```python
from build123d import *

# Parameters (mm, degrees)
SKETCH1_W                    = 50
SKETCH1_H                    = 150
BASE_FLANGE1_DEPTH           = 6
EDGE_FLANGE1_STRIP_W         = 36
EDGE_FLANGE1_STRIP_H         = 6
EDGE_FLANGE1_STRIP_CUT_DEPTH = 150
EDGE_FLANGE1_DEPTH           = 150
SKETCH9_R                    = 4
CUT_EXTRUDE1_DEPTH           = 6
CUT_EXTRUDE2_DEPTH           = 10
FILLET1_R                    = 5
SKETCH11_W                   = 20
SKETCH11_H                   = 80
SKETCH11_W_2                 = 70
SKETCH11_R                   = 4
SKETCH11_R_2                 = 20
CUT_EXTRUDE5_DEPTH           = 10


# Sheet-metal steps are written as plain solids
with BuildPart() as part:
    # Sketch1 → Base-Flange1 (new body)
    with BuildSketch(Plane.XY):
        with Locations((25, 75)):
            Rectangle(SKETCH1_W, SKETCH1_H)
    extrude(amount=-BASE_FLANGE1_DEPTH)

    # Edge-Flange1 strip (across the edge) → Edge-Flange1 strip cut (cut)
    with BuildSketch(Plane(origin=(50, 0, 0), x_dir=(-1, 0, 0), z_dir=(0, 1, 0))):
        with Locations((-6, -3)):
            Rectangle(EDGE_FLANGE1_STRIP_W, EDGE_FLANGE1_STRIP_H)
    extrude(amount=EDGE_FLANGE1_STRIP_CUT_DEPTH, mode=Mode.SUBTRACT)

    # Edge-Flange1 section (across the edge) → Edge-Flange1 (add)
    with BuildSketch(Plane(origin=(50, 0, 0), x_dir=(-1, 0, 0), z_dir=(0, 1, 0))):
        with BuildLine():
            Line((0, 6), (0, 144))
            Line((0, 144), (6, 144))
            Line((6, 144), (6, 6))
            ThreePointArc((6, 6), (7.757359313, 1.757359313), (12, 0))
            Line((12, 0), (12, -6))
            ThreePointArc((12, -6), (3.514718626, -2.485281374), (0, 6))
        make_face()
    extrude(amount=EDGE_FLANGE1_DEPTH)

    # Sketch9 → Cut-Extrude1 (cut)
    with BuildSketch(Plane.XY):
        with Locations((6.5, 135)):
            Circle(SKETCH9_R)
        with Locations((31.5, 135)):
            Circle(SKETCH9_R)
        with Locations((6.5, 15)):
            Circle(SKETCH9_R)
        with Locations((31.5, 15)):
            Circle(SKETCH9_R)
    extrude(amount=-CUT_EXTRUDE1_DEPTH, mode=Mode.SUBTRACT)

    # Sketch10 → Cut-Extrude2 (cut)
    with BuildSketch(Plane(origin=(50, 0, 0), x_dir=(0, 0, -1), z_dir=(1, 0, 0))):
        with BuildLine():
            Line((-130, 139), (-20, 139))
            ThreePointArc((-20, 139), (-16, 135), (-20, 131))
            Line((-20, 131), (-130, 131))
            ThreePointArc((-130, 131), (-134, 135), (-130, 139))
        make_face()
        with BuildLine():
            Line((-130, 11), (-20, 11))
            ThreePointArc((-20, 11), (-16, 15), (-20, 19))
            Line((-20, 19), (-130, 19))
            ThreePointArc((-130, 19), (-134, 15), (-130, 11))
        make_face()
    extrude(amount=-CUT_EXTRUDE2_DEPTH, mode=Mode.SUBTRACT)

    # Fillet1
    fillet1_edges = [part.edges().sort_by_distance(p)[0] for p in [
        (47, 0, 144),
        (47, 150, 144),
        (0, 0, -3),
        (0, 150, -3),
    ]]
    fillet(fillet1_edges, radius=FILLET1_R)

    # Sketch11 → Cut-Extrude5 (cut)
    # profile 1 of 6: a face of its own
    with BuildSketch(Plane(origin=(50, 0, 0), x_dir=(0, 0, -1), z_dir=(1, 0, 0))):
        with Locations((-117.5, 75)):
            Rectangle(SKETCH11_W, SKETCH11_H)
    # profile 2 of 6: a face of its own
    with BuildSketch(Plane(origin=(50, 0, 0), x_dir=(0, 0, -1), z_dir=(1, 0, 0))):
        with Locations((-27.5, 75)):
            Rectangle(SKETCH11_W, SKETCH11_H)
    # profile 3 of 6: a face of its own
    with BuildSketch(Plane(origin=(50, 0, 0), x_dir=(0, 0, -1), z_dir=(1, 0, 0))):
        with Locations((-72.5, 75)):
            Rectangle(SKETCH11_W_2, SKETCH11_H)
        with Locations((-97.5, 50)):
            Circle(SKETCH11_R, mode=Mode.SUBTRACT)
        with Locations((-47.5, 50)):
            Circle(SKETCH11_R, mode=Mode.SUBTRACT)
        with Locations((-72.5, 75)):
            Circle(SKETCH11_R_2, mode=Mode.SUBTRACT)
        with Locations((-97.5, 100)):
            Circle(SKETCH11_R, mode=Mode.SUBTRACT)
        with Locations((-47.5, 100)):
            Circle(SKETCH11_R, mode=Mode.SUBTRACT)
    # profile 4 of 6: a face of its own
    with BuildSketch(Plane(origin=(50, 0, 0), x_dir=(0, 0, -1), z_dir=(1, 0, 0))):
        with Locations((-72.5, 75)):
            Circle(SKETCH11_R_2)
    # profile 5 of 6: a face of its own
    with BuildSketch(Plane(origin=(50, 0, 0), x_dir=(0, 0, -1), z_dir=(1, 0, 0))):
        with Locations((-47.5, 50)):
            Circle(SKETCH11_R)
    # profile 6 of 6: a face of its own
    with BuildSketch(Plane(origin=(50, 0, 0), x_dir=(0, 0, -1), z_dir=(1, 0, 0))):
        with Locations((-47.5, 100)):
            Circle(SKETCH11_R)
    extrude(amount=-CUT_EXTRUDE5_DEPTH, mode=Mode.SUBTRACT)


with BuildPart() as cut_extrude5_kept_piece:
    # of the separate pieces the step leaves, the one the design keeps (cut_extrude5_pieces_kept)
    add(part.part.solids().sort_by_distance((0, 5, 0))[0])


solid = cut_extrude5_kept_piece.part
```
The listing builds one solid part. Answer for the finished solid, in the listing's coordinates (mm). A direction names the side the tool comes from. Give positions to 0.01 mm unless a question says otherwise; leave off trailing zeros. Order: outer loops, then holes, each group sorted by start corner. A loop starts at its lowest first (then second) coordinate and runs counter-clockwise, first axis right, second up. Notation, with made-up numbers: (-38.75, 55) -> (10.25, 55) arc R29 cw to (10.25, 84) -> close; hole circle Ø9 at (18, -25.5). An arc over 180 degrees is marked (long way). Write each question's results on one line, items separated by ' | '.
Q1. The part is cut by section A-A, the plane x = 31.5. Give the vertices of the cut face in (y, z), and give its area (3 significant figures).
Checked values:
outline: (0, -6) -> (11, -6) -> (11, 0) -> (0, 0) -> close; (19, -6) -> (131, -6) -> (131, 0) -> (19, 0) -> close; (139, -6) -> (150, -6) -> (150, 0) -> (139, 0) -> close | area: 804 mm^2
Q2. Each of these flat-tipped pins is pushed along its axis until it touches: P1, Ø1.5, axis at x = 12, y = 91.5, coming from the +Z side; P2, Ø3, axis at x = 46.5, y = 55.5, coming from the -Z side. Where does it stop, or does it pass through?
Checked values:
P1: stops at z = 0 | P2: stops at z = -3.75
Q3. The part is cut by section B-B, the plane y = 69. Give the vertices of the cut face in (x, z).
Checked values:
outline: (0, -6) -> (38, -6) arc R12 ccw to (50, 6) -> (50, 17.5) -> (44, 17.5) -> (44, 6) arc R6 cw to (38, 0) -> (0, 0) -> close; (44, 127.5) -> (50, 127.5) -> (50, 144) -> (44, 144) -> close
Q4. The part is cut by section D-D, the plane y = 15. Give the vertices of the cut face in (x, z), and give its area (3 significant figures).
Checked values:
outline: (0, -6) -> (2.5, -6) -> (2.5, 0) -> (0, 0) -> close; (10.5, -6) -> (27.5, -6) -> (27.5, 0) -> (10.5, 0) -> close; (35.5, -6) -> (38, -6) arc R12 ccw to (50, 6) -> (50, 16) -> (44, 16) -> (44, 6) arc R6 cw to (38, 0) -> (35.5, 0) -> close; (44, 134) -> (50, 134) -> (50, 144) -> (44, 144) -> close | area: 337 mm^2
Q5. Which of the six approach directions +Z, -Z, +X, -X, +Y, -Y give full straight-line access (tool end or side, diameter ignored) to faces 1 (the face through (2, 1, -3)), 2 (the face through (47, 135, 134))?
Checked values:
face 1: +Z, -Z, -X, -Y | face 2: +X, -X
Q6. Determine the mould class of faces 3 (the face through (47, 19, 74)), 4 (the face through (47, 149, 142)), 5 (the face through (5.979, 18.966, -2.958)), 6 (the face through (47, 74, 127.5)) for opening direction Z: pulls with the +Z half, pulls with the -Z half, needs draft (parallel to the pull), parting line crosses it, or undercut.
Checked values:
face 3: undercut | face 4: pulls with the +Z half | face 5: needs draft | face 6: undercut
Q7. The part is cut by section C-C, the plane z = 26. Give the vertices of the cut face in (x, y), and give its area (3 significant figures).
Checked values:
outline: (44, 0) -> (50, 0) -> (50, 11) -> (44, 11) -> close; (44, 19) -> (50, 19) -> (50, 35) -> (44, 35) -> close; (44, 115) -> (50, 115) -> (50, 131) -> (44, 131) -> close; (44, 139) -> (50, 139) -> (50, 150) -> (44, 150) -> close | area: 324 mm^2
Q8. Straight lines are drawn through the part: probe 1 along Y at (x, z) = (6, -4); probe 2 along X at (y, z) = (143.5, 104.5); probe 3 along Z at (x, y) = (14.5, 89). For each, find the intervals that lie inside material, in ascending order. Write a range as from..to.
Checked values:
probe 1: y = 0..11.03, 18.97..131.03, 138.97..150 | probe 2: x = 44..50 | probe 3: z = -6..0
